```python
from build123d import *

# Parameters (mm, degrees)
F0_W       = 6.35
F0_H       = 56.2863781022
F1_DEPTH   = 57.15
F0_R       = 3.2639
F0_R_2     = 2.0955
F2_DEPTH   = 6.35
F4_SIZE2   = 1.27
F4_SIZE    = 1.5875
F4_2_SIZE2 = 1.27
F4_2_SIZE  = 1.5875
F4_3_SIZE2 = 1.27
F4_3_SIZE  = 1.5875
F4_4_SIZE2 = 1.27
F4_4_SIZE  = 1.5875
F5_R       = 1.6002
F6_SIZE    = 0.508
F7_R       = 3.2639
F7_R_2     = 2.0955
F8_DEPTH   = 114.9842375546
F9_SIZE    = 0.508


# Not quite as in the source:
# - a feature names something its author has since deleted; it is built from what else it names


with BuildPart() as f1:
    # F0 (on Front) → F1 (new body)
    with BuildSketch(Plane.XZ):
        with Locations((-35.56, 0)):
            Rectangle(F0_W, F0_H)
    extrude(amount=F1_DEPTH)



with BuildPart() as f1b:
    # F0 (on Front) → F1, piece 2 (new body)
    with BuildSketch(Plane.XZ):
        with Locations((35.56, 0)):
            Rectangle(F0_W, F0_H)
    extrude(amount=F1_DEPTH)


with BuildPart() as f1_1:
    add(f1.part)

    add(f1b.part)  # F2 merges F1b
    # F0 (on Front) → F2 (join)
    with BuildSketch(Plane.XZ):
        Polygon((-76.249649699, 28.1431890511), (-76.2, -28.1431890511), (-38.735, -28.1431890511), (-38.735, 28.1431890511), align=None)
        with Locations((-66.7125248495, -9.0931890511)):
            Circle(F0_R, mode=Mode.SUBTRACT)
        with Locations((-48.26, -9.0424341398)):
            Circle(F0_R, mode=Mode.SUBTRACT)
        with Locations((-66.7125248495, 14.4018109489)):
            Circle(F0_R, mode=Mode.SUBTRACT)
        with Locations((-48.26, 14.4525658602)):
            Circle(F0_R, mode=Mode.SUBTRACT)
        Polygon((-32.385, 28.1431890511), (-32.385, -28.1431890511), (0, -28.1431890511), (32.385, -28.1431890511), (32.385, 28.1431890511), (0, 28.1431890511), align=None)
        with Locations((-24.13, -21.0311890511)):
            Circle(F0_R_2, mode=Mode.SUBTRACT)
        with Locations((24.13, -21.0311890511)):
            Circle(F0_R_2, mode=Mode.SUBTRACT)
        with Locations((-24.13, 21.3106109489)):
            Circle(F0_R_2, mode=Mode.SUBTRACT)
        with Locations((24.13, 21.3106109489)):
            Circle(F0_R_2, mode=Mode.SUBTRACT)
        Polygon((38.735, 28.1431890511), (38.735, -28.1431890511), (76.2, -28.1431890511), (76.249649699, 28.1431890511), align=None)
        with Locations((48.26, -9.0424341398)):
            Circle(F0_R, mode=Mode.SUBTRACT)
        with Locations((66.7125248495, -9.0931890511)):
            Circle(F0_R, mode=Mode.SUBTRACT)
        with Locations((48.26, 14.4525658602)):
            Circle(F0_R, mode=Mode.SUBTRACT)
        with Locations((66.7125248495, 14.4018109489)):
            Circle(F0_R, mode=Mode.SUBTRACT)
    extrude(amount=F2_DEPTH)

    # F3: union 

    # F4
    f4_edges = [f1_1.edges().sort_by_distance(p)[0] for p in [
        (22.0345, 0, 21.310611),
    ]]
    f4_side = f1_1.faces().sort_by_distance((22.0345, -3.175, 21.310611))[0]
    chamfer(f4_edges, length=F4_SIZE, length2=F4_SIZE2, reference=f4_side)

    # F4#2
    f4_2_edges = [f1_1.edges().sort_by_distance(p)[0] for p in [
        (-26.2255, 0, 21.310611),
    ]]
    f4_2_side = f1_1.faces().sort_by_distance((-26.2255, -3.175, 21.310611))[0]
    chamfer(f4_2_edges, length=F4_2_SIZE, length2=F4_2_SIZE2, reference=f4_2_side)

    # F4#3
    f4_3_edges = [f1_1.edges().sort_by_distance(p)[0] for p in [
        (22.0345, 0, -21.031189),
    ]]
    f4_3_side = f1_1.faces().sort_by_distance((22.0345, -3.175, -21.031189))[0]
    chamfer(f4_3_edges, length=F4_3_SIZE, length2=F4_3_SIZE2, reference=f4_3_side)

    # F4#4
    f4_4_edges = [f1_1.edges().sort_by_distance(p)[0] for p in [
        (-26.2255, 0, -21.031189),
    ]]
    f4_4_side = f1_1.faces().sort_by_distance((-26.2255, -3.175, -21.031189))[0]
    chamfer(f4_4_edges, length=F4_4_SIZE, length2=F4_4_SIZE2, reference=f4_4_side)

    # F5
    f5_edges = [f1_1.edges().sort_by_distance(p)[0] for p in [
        (76.24965, -3.175, 28.143189),
        (-76.24965, -3.175, 28.143189),
        (76.2, -3.175, -28.143189),
        (-76.2, -3.175, -28.143189),
        (-35.56, -57.15, 28.143189),
        (-35.56, -57.15, -28.143189),
        (35.56, -57.15, 28.143189),
        (35.56, -57.15, -28.143189),
    ]]
    fillet(f5_edges, radius=F5_R)

    # F6
    f6_edges = [f1_1.edges().sort_by_distance(p)[0] for p in [
        (63.448625, 0, 14.401811),
        (44.9961, 0, 14.452566),
        (63.448625, 0, -9.093189),
        (44.9961, 0, -9.042434),
        (-51.5239, 0, 14.452566),
        (-69.976425, 0, 14.401811),
        (-69.976425, 0, -9.093189),
        (-51.5239, 0, -9.042434),
        (76.224824, 0, -0.001412),
        (-56.691519, -6.35, 28.143189),
        (0, -6.35, 28.143189),
        (76.224824, -6.35, -0.001412),
        (0, -6.35, -28.143189),
        (32.385, -30.9499, -28.143189),
        (35.56, -55.5498, -28.143189),
        (38.735, -30.9499, -28.143189),
        (-32.385, -30.9499, -28.143189),
        (56.668105, -6.35, -28.143189),
        (-35.56, -55.5498, -28.143189),
        (74.601211, -3.175, -28.143189),
        (-38.735, -30.9499, -28.143189),
        (0, 0, -28.143189),
        (-56.668105, -6.35, -28.143189),
        (-74.601211, -3.175, -28.143189),
        (56.691519, -6.35, 28.143189),
        (-69.976425, -6.35, 14.401811),
        (-51.5239, -6.35, 14.452566),
        (-69.976425, -6.35, -9.093189),
        (-51.5239, -6.35, -9.042434),
        (-26.2255, -6.35, 21.310611),
        (22.0345, -6.35, 21.310611),
        (-26.2255, -6.35, -21.031189),
        (22.0345, -6.35, -21.031189),
        (44.9961, -6.35, 14.452566),
        (63.448625, -6.35, 14.401811),
        (44.9961, -6.35, -9.042434),
        (63.448625, -6.35, -9.093189),
    ]]
    chamfer(f6_edges, length=F6_SIZE)

    # F7 (on face) → F8 (cut, through all)
    with BuildSketch(Plane.YZ.offset(38.735)):
        with Locations((-47.879, 4.3688109489)):
            Circle(F7_R)
        with Locations((-16.129, 4.3688109489)):
            Circle(F7_R)
        with Locations((-47.879, 21.3106109489)):
            Circle(F7_R_2)
        with Locations((-16.129, 21.3106109489)):
            Circle(F7_R_2)
        with Locations((-32.004, 21.3106109489)):
            Circle(F7_R_2)
        with Locations((-47.879, -21.0311890511)):
            Circle(F7_R_2)
        with Locations((-32.004, -21.0311890511)):
            Circle(F7_R_2)
        with Locations((-16.129, -21.0311890511)):
            Circle(F7_R_2)
        with Locations((-32.004, 4.3688109489)):
            Circle(F7_R)
    extrude(amount=-F8_DEPTH, mode=Mode.SUBTRACT)

    # F9
    f9_edges = [f1_1.edges().sort_by_distance(p)[0] for p in [
        (38.735, -51.1429, 4.368811),
        (38.735, -19.3929, 4.368811),
        (32.385, -51.1429, 4.368811),
        (32.385, -19.3929, 4.368811),
        (-32.385, -51.1429, 4.368811),
        (-32.385, -19.3929, 4.368811),
        (-38.735, -51.1429, 4.368811),
        (-38.735, -19.3929, 4.368811),
        (38.735, -49.9745, 21.310611),
        (38.735, -34.0995, 21.310611),
        (38.735, -18.2245, 21.310611),
        (38.735, -49.9745, -21.031189),
        (38.735, -34.0995, -21.031189),
        (38.735, -18.2245, -21.031189),
        (38.735, -35.2679, 4.368811),
        (32.385, -49.9745, 21.310611),
        (32.385, -49.9745, -21.031189),
        (32.385, -34.0995, 21.310611),
        (32.385, -35.2679, 4.368811),
        (32.385, -18.2245, 21.310611),
        (32.385, -34.0995, -21.031189),
        (32.385, -18.2245, -21.031189),
        (-32.385, -49.9745, -21.031189),
        (-32.385, -49.9745, 21.310611),
        (-32.385, -34.0995, -21.031189),
        (-32.385, -18.2245, -21.031189),
        (-32.385, -35.2679, 4.368811),
        (-32.385, -34.0995, 21.310611),
        (-32.385, -18.2245, 21.310611),
        (-38.735, -49.9745, 21.310611),
        (-38.735, -49.9745, -21.031189),
        (-38.735, -34.0995, 21.310611),
        (-38.735, -35.2679, 4.368811),
        (-38.735, -18.2245, 21.310611),
        (-38.735, -34.0995, -21.031189),
        (-38.735, -18.2245, -21.031189),
    ]]
    chamfer(f9_edges, length=F9_SIZE)


solid = f1_1.part
```
Build history of the part. All positions in model axes, mm. A direction names the side the tool comes from. Round coordinates to 2 decimals unless told otherwise and drop trailing zeros. Write each loop counter-clockwise with the first axis right and the second up, starting at its lowest first coordinate (ties: lowest second). Pieces come first, ordered by that corner, then holes. Notation, with made-up numbers: (39, 27) - (98, 27) arc R14 ccw to (98, 34) - close; hole circle Ø8 at (82, 17.25). An arc over 180 degrees is marked (long way). Answer as CSV lines item,"result".
Q1. Cut at B-B (y = -10). Write the cut outline in (x, z) (3 decimals), and give its area (3 significant figures).
Report:
outline,"(-38.735, -27.635) - (-38.227, -28.143) - (-32.893, -28.143) - (-32.385, -27.635) - (-32.385, 27.635) - (-32.893, 28.143) - (-38.227, 28.143) - (-38.735, 27.635) - close; (32.385, -27.635) - (32.893, -28.143) - (38.227, -28.143) - (38.735, -27.635) - (38.735, 27.635) - (38.227, 28.143) - (32.893, 28.143) - (32.385, 27.635) - close"
area,"714 mm^2"
Q2. Cut at D-D (x = 24.13). Write the cut outline in (y, z), and give its area (3 significant figures).
Report:
outline,"(-6.35, -27.64) - (-5.84, -28.14) - (-0.51, -28.14) - (0, -27.64) - (0, -24.4) - (-1.59, -23.13) - (-5.84, -23.13) - (-6.35, -23.63) - close; (-6.35, -18.43) - (-5.84, -18.94) - (-1.59, -18.94) - (0, -17.67) - (0, 17.95) - (-1.59, 19.22) - (-5.84, 19.22) - (-6.35, 18.71) - close; (-6.35, 23.91) - (-5.84, 23.41) - (-1.59, 23.41) - (0, 24.68) - (0, 27.64) - (-0.51, 28.14) - (-5.84, 28.14) - (-6.35, 27.64) - close"
area,"299 mm^2"
Q3. Cut at C-C (x = 56). Write the cut outline in (y, z), and give its area (3 significant figures).
Report:
outline,"(-6.35, -27.64) - (-5.84, -28.14) - (-0.51, -28.14) - (0, -27.64) - (0, 27.64) - (-0.51, 28.14) - (-5.84, 28.14) - (-6.35, 27.64) - close"
area,"357 mm^2"
Q4. Pull direction Y, two halves, no side cores. Call faces 1 (the cylindrical face through (25.097, -3.685, 19.452)), 2 (the flat face through (-36, -57.15, 0)), 3 (the cylindrical face through (-35.523, -17.792, 20.036)): +Y half, -Y half, draft (parallel to the pull), parting line (faces both ways), or undercut.
Report:
face 1,"draft"
face 2,"-Y half"
face 3,"undercut"
Q5. Drop flat-ended pins along their axis: pin 1 (1 mm diameter, centred on y = -48, z = 9, fed in from +X) (3 decimals); pin 2 (1.5 mm diameter, centred on x = -4, z = -3.5, fed in from -Y); pin 3 (5.5 mm diameter, centred on x = 24.13, z = 21.31, fed in from +Y). Give the stop position or say it passes through.
Report:
pin 1,"stops at x = 38.735"
pin 2,"stops at y = -6.35"
pin 3,"stops at y = -0.77"
Q6. Cut at A-A (x = -48.26). Write the cut outline in (y, z).
Report:
outline,"(-6.35, -27.64) - (-5.84, -28.14) - (-0.51, -28.14) - (0, -27.64) - (0, -12.81) - (-0.51, -12.31) - (-5.84, -12.31) - (-6.35, -12.81) - close; (-6.35, -5.27) - (-5.84, -5.78) - (-0.51, -5.78) - (0, -5.27) - (0, 10.68) - (-0.51, 11.19) - (-5.84, 11.19) - (-6.35, 10.68) - close; (-6.35, 18.22) - (-5.84, 17.72) - (-0.51, 17.72) - (0, 18.22) - (0, 27.64) - (-0.51, 28.14) - (-5.84, 28.14) - (-6.35, 27.64) - close"
Q7. Drill centre lines: probe 1 along Z at (x, y) = (48.26, -4); probe 2 along X at (y, z) = (-22.5, -24) (3 decimals); probe 3 along Y at (x, z) = (-53.5, -6.5). Where is each one in solid material? Low to high. Write a range as [from, to].
Report:
probe 1,"z = [-28.14, -12.31], [-5.78, 11.19], [17.72, 28.14]"
probe 2,"x = [-38.735, -32.385], [32.385, 38.735]"
probe 3,"y = [-6.35, 0]"
Q8. Tool access for faces 4 (the cylindrical face through (35.597, -49.542, 20.036)), 5 (the flat face through (-32.385, -31, 0)): list every direction of +Z, -Z, +X, -X, +Y, -Y with a clear straight run to the whole face (end or side of a thin tool).
Report:
face 4,"+X, -X"
face 5,"+Z, -Z, -Y"
